Here's how the part is built. I have some questions about the finished solid (model axes, mm). Face numbers are marked on the shaded views. Give positions to 0.01 mm unless a question says otherwise; leave off trailing zeros. Loops run counter-clockwise (first coordinate to the right, second up) from the corner with the lowest first, then second, coordinate; pieces in that order, holes last. Notation, with made-up numbers: (66, 28.5) - (115, 28.5) arc R16 ccw to (115, 55.5) - close; hole circle Ø10 at (75, 57.25). An arc over 180 degrees is marked (long way). One line per item, written item: value. Start each with the question number.
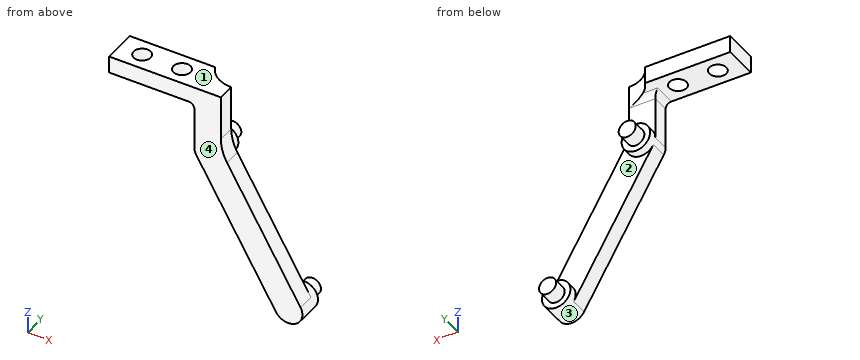
```python
from build123d import *

# Parameters (mm, degrees)
BOSS_EXTRUDE1_DEPTH = 3
SKETCH1_4_R         = 2.5000000000000004
SKETCH1_4_R_2       = 1.5
SKETCH1_4_R_3       = 2.500000000000002
SKETCH1_4_R_4       = 1.5000000000000009
BOSS_EXTRUDE2_DEPTH = 4.5
SKETCH1_5_R         = 1.5
SKETCH1_5_R_2       = 1.5000000000000009
BOSS_EXTRUDE3_DEPTH = 7
BOSS_EXTRUDE4_DEPTH = 15
SKETCH4_R           = 1.4999999999999987
SKETCH4_R_2         = 1.5000000000000007
CUT_EXTRUDE1_DEPTH  = 20
FILLET1_R           = 5
FILLET2_R           = 1
FILLET3_R           = 8


with BuildPart() as part:
    # Sketch1 → Boss-Extrude1 (new body)
    with BuildSketch(Plane(origin=(0, 0, 0), x_dir=(1, 0, 0), z_dir=(0, 1, 0))):
        with BuildLine():
            Line((11.840552747753916, 25.259677563810218), (-2.159447252246084, 1.2596775638102156))
            ThreePointArc((-2.1594472522460837, 1.2596775638102162), (0.6524499480361662, 2.413360533635123), (2.5000000000000004, 0))
            ThreePointArc((2.5000000000000004, -6.1e-16), (2.413360533635123, -0.6524499480361662), (2.159447252246083, -1.2596775638102173))
            Line((2.159447252246083, -1.2596775638102156), (16.15944725224609, 22.740322436189782))
            ThreePointArc((16.159447252246085, 22.740322436189782), (12.740322436189784, 21.840552747753915), (11.840552747753918, 25.259677563810218))
        make_face()
        Polygon((2.1594472522460837, -3), (-2.5, -3), (-2.499999999999999, -11.259677563810214), (2.1594472522460846, -11.259677563810214), align=None)
        with BuildLine():
            ThreePointArc((2.159447252246083, -1.2596775638102173), (-0.6524499480361661, -2.413360533635123), (-2.5000000000000004, 3.1e-16))
            Line((-2.5000000000000004, 0), (-2.5, -3))
            Line((-2.5, -3), (2.1594472522460837, -3))
            Line((2.1594472522460832, -3), (2.159447252246083, -1.2596775638102156))
        make_face()
    extrude(amount=BOSS_EXTRUDE1_DEPTH)

    # Sketch1<4> → Boss-Extrude2 (add)
    # profile 1 of 2: a face of its own
    with BuildSketch(Plane(origin=(0, 0, 0), x_dir=(1, 0, 0), z_dir=(0, 1, 0))):
        with Locations(Location((0, 0, 0), (0, 0, 149.743562836))):
            Circle(SKETCH1_4_R)
        with Locations(Location((0, 0, 0), (0, 0, 270))):
            Circle(SKETCH1_4_R_2, mode=Mode.SUBTRACT)
    # profile 2 of 2: a face of its own
    with BuildSketch(Plane(origin=(0, 0, 0), x_dir=(1, 0, 0), z_dir=(0, 1, 0))):
        with Locations(Location((14.000000000000002, 24, 0), (0, 0, 149.743562836))):
            Circle(SKETCH1_4_R_3)
        with Locations(Location((14.000000000000002, 24, 0), (0, 0, 270))):
            Circle(SKETCH1_4_R_4, mode=Mode.SUBTRACT)
    extrude(amount=BOSS_EXTRUDE2_DEPTH)

    # Sketch1<5> → Boss-Extrude3 (add)
    with BuildSketch(Plane(origin=(0, 0, 0), x_dir=(1, 0, 0), z_dir=(0, 1, 0))):
        with Locations(Location((0, 0, 0), (0, 0, 270))):
            Circle(SKETCH1_5_R)
        with Locations(Location((14.000000000000002, 24, 0), (0, 0, 270))):
            Circle(SKETCH1_5_R_2)
    extrude(amount=BOSS_EXTRUDE3_DEPTH)

    # Sketch3 → Boss-Extrude4 (add)
    with BuildSketch(Plane.ZY.offset(2.5000000000000004)):
        Polygon((11.259677563810214, 0), (8.259677563810214, -3.7e-16), (8.259677563810214, 6), (11.259677563810214, 6.000000000000001), align=None)
    extrude(amount=BOSS_EXTRUDE4_DEPTH)

    # Sketch4 → Cut-Extrude1 (cut)
    with BuildSketch(Plane(origin=(9.5e-16, 0, 8.259677563810214), x_dir=(-1, 0, 1.2e-16), z_dir=(-1.2e-16, 0, -1))):
        with Locations((6.500000000000001, 2.999999999999998)):
            Circle(SKETCH4_R)
        with Locations((13.499999999999998, 2.9999999999999996)):
            Circle(SKETCH4_R_2)
    extrude(amount=-CUT_EXTRUDE1_DEPTH, mode=Mode.SUBTRACT)

    # Fillet1
    # the kernel refuses this fillet: 5 mm, written as the material it adds along each edge
    with BuildSketch(Plane(origin=(-2.499999999999999, 3, 11.259677563810214), x_dir=(1, 0, -1.6e-16), z_dir=(-1.6e-16, 0, -1))) as fillet1_piece_1:
        with BuildLine():
            CenterArc((4.582575694955841, -5), FILLET1_R, 90, 66.42182152179817)
            Line((8.9e-16, -3), (0, 0))
            Line((0, 0), (4.582575694955841, 0))
        make_face()
    extrude(amount=3)

    # Fillet2
    fillet2_edges = [part.edges().sort_by_distance(p)[0] for p in [
        (-2.4999999999999996, 1.4999999999999998, 8.259677563810214),
        (-0.20871215252200015, 3, 8.25967756381),
    ]]
    fillet(fillet2_edges, radius=FILLET2_R)

    # Fillet3
    fillet3_edges = [part.edges().sort_by_distance(p)[0] for p in [
        (2.159447252246083, 1.5, 1.2596775638102164),
    ]]
    fillet(fillet3_edges, radius=FILLET3_R)


solid = part.part
```
(1) Will these pins go through, and if not, where does the flat tip stop? pin 1 (2.5 mm diameter, centred on x = -13.5, y = 3, fed in from -Z); pin 2 (2.5 mm diameter, centred on y = 2, z = 7.5, fed in from +X); pin 3 (4 mm diameter, centred on y = 1.5, z = 3.5, fed in from +X); pin 4 (2.5 mm diameter, centred on x = -6.5, z = 10, fed in from +Y).
(2) Please list where these lines run through material, in increasing order: probe 1 along Y at (x, z) = (-6.5, 9.25); probe 2 along X at (y, z) = (4, 2); probe 3 along Y at (x, z) = (-6, 10). Write a range as from..to.
(3) If we section it at A-A on x = -13.5: List the corners of the cut face in (y, z) for me, plus the area to 3 significant figures.
(4) If we mould it in two halves opening along Z, with no side actions, what happens to the marked faces 1, 2, 3 and 4? For each: pulls with the +Z half, pulls with the -Z half, needs draft (parallel to the pull), parting line crosses it, or undercut.
(5) If we section it at B-B on y = 1: List the corners of the cut face in (x, z) for me.
(6) If we section it at C-C on x = -9: List the corners of the cut face in (y, z) for me.
(7) If we section it at D-D on z = -24: List the corners of the cut face in (x, y) for me, plus the area to 3 significant figures.
Found:
1. pin 1: through
1. pin 2: x = 2.16
1. pin 3: x = 2.39
1. pin 4: y = 6
2. probe 1: 0..1.5, 4.5..6
2. probe 2: -1.5..1.5
2. probe 3: 0..1.59, 4.41..6
3. outline: (0, 8.26) - (1.5, 8.26) - (1.5, 11.26) - (0, 11.26) - close; (4.5, 8.26) - (6, 8.26) - (6, 11.26) - (4.5, 11.26) - close
3. area: 9.00 mm^2
4. face 1: pulls with the +Z half
4. face 2: undercut
4. face 3: parting line crosses it
4. face 4: needs draft
5. outline: (-17.5, 8.26) - (-3.5, 8.26) arc R1 cw to (-2.5, 7.26) - (-2.5, 0) arc R2.5 ccw to (-2.16, -1.26) - (11.84, -25.26) arc R2.5 ccw to (16.16, -22.74) - (3.25, -0.61) arc R8 cw to (2.16, 3.42) - (2.16, 11.26) - (-17.5, 11.26) - close
6. outline: (0, 8.26) - (6, 8.26) - (6, 11.26) - (0, 11.26) - close
7. outline: (11.11, 0) - (16.5, 0) - (16.5, 4.5) - (15.5, 4.5) - (15.5, 7) - (12.5, 7) - (12.5, 4.5) - (11.5, 4.5) - (11.5, 3) - (11.11, 3) - close
7. area: 31.2 mm^2
